Build history of the part. All positions in model axes, mm. Face numbers are marked on the shaded views. A direction names the side the tool comes from. Coordinates: 2 decimals unless noted, no trailing zeros. Loops run counter-clockwise (first coordinate to the right, second up) from the corner with the lowest first, then second, coordinate; pieces in that order, holes last.
(1) Slice it at A-A (z = -5). Give the cut face in (x, y), and give its area (3 significant figures).
(2) Flat gauge pins, fed straight in: P1, Ø4, axis at y = 5.5, z = -4, coming from the -X side; P2, Ø6, axis at x = -6, z = 15, coming from the -Y side; P3, Ø3, axis at x = 3, z = 14.5, coming from the -Y side. Where does each tip first touch, or does it go through?
(3) Slice it at B-B (z = 3). Give the cut face in (x, y).
(4) Wall check: L1, parallel to X at y = -2.5, z = 10.25; L2, parallel to Z at x = -5.5, y = -5.5; L3, parallel to Z at x = -3.5, y = 0.75. Give the ranges that are in metal, low to high.
(5) Tool access for the marked faces 1 and 2: list every direction of +Z, -Z, +X, -X, +Y, -Y with a clear straight run to the whole face (end or side of a thin tool).
from build123d import *

# Parameters (mm, degrees)
F0_R        = 6.85
F1_DEPTH    = 8
F4_R        = 7.62
F5_S5_R     = 6.85
F5_T6_DEPTH = 16
F6_R        = 2.54


# Not quite as in the source:
# - a fillet or chamfer that OpenCascade refuses, or shapes differently, is made with other operations: its cross-section is extruded or revolved along the edge and cut away or added


with BuildPart() as f1:
    # F0 (on Top) → F1 (new body)
    with BuildSketch(Plane.XY):
        Circle(F0_R)
    extrude(amount=-F1_DEPTH)

    # F2 (on Front) → F3 (revolve)
    with BuildSketch(Plane.XZ):
        Polygon((-10.0059127435, 0), (0, 0), (0, 20), (-7.62, 20), align=None)
    revolve(axis=Axis((0, 0, 10), (0, 0, 1)))

    # F4
    f4_edges = [f1.edges().sort_by_distance(p)[0] for p in [
        (7.62, 0, 20),
    ]]
    fillet(f4_edges, radius=F4_R)

    # F5: chamfer of 5.08 on 1 edges, made by hand


with BuildPart() as f5_tool2:
    # F5_s3 → F5_t4 (revolve)
    with BuildSketch(Plane.XZ):
        Polygon((-9.4041577027, 5.0442334275), (-4.9259127435, 0), (-10.0059127435, 0), align=None)
    revolve(axis=Axis((0, 0, 0), (0, 0, 1)))

    # F5_s5 → F5_t6 (cut, symmetric)
    with BuildSketch(Plane.XY.offset(2.5)):
        Circle(F5_S5_R)
    extrude(amount=F5_T6_DEPTH, both=True, mode=Mode.SUBTRACT)


with BuildPart() as f1_1:
    add(f1.part)

    # F5_t1: cut F5_tool2
    add(f5_tool2.part, mode=Mode.SUBTRACT)

    # F6
    f6_edges = [f1_1.edges().sort_by_distance(p)[0] for p in [
        (9.404158, 0, 5.044233),
    ]]
    fillet(f6_edges, radius=F6_R)


solid = f1_1.part
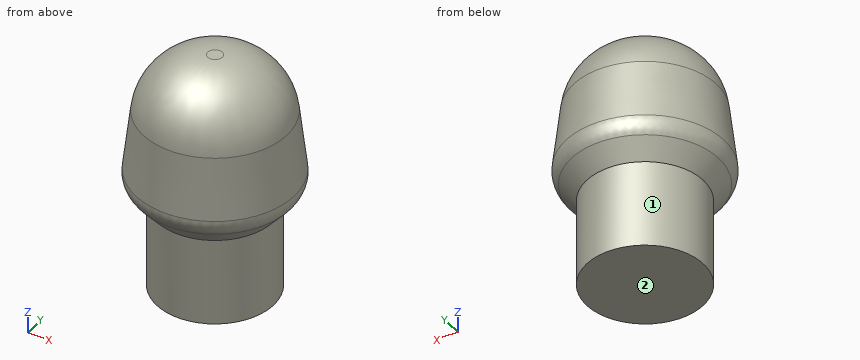
Response values:
1. outline: circle Ø13.7 at (0, 0)
1. area: 147 mm2
2. P1: stops at x = -5.89
2. P2: stops at y = -7.68
2. P3: stops at y = -8.18
3. outline: circle Ø15.18 at (0, 0)
4. L1: x = -8.42 to 8.42
4. L2: z = 3.21 to 15.56
4. L3: z = -8 to 19.5
5. face 1: -Z
5. face 2: -Z, +X, -X, +Y, -Y
